Can you work these out from the model? Positions are in its coordinate system, mm. Face numbers are marked on the shaded views. A direction names the side the tool comes from. Round coordinates to 2 decimals unless told otherwise and drop trailing zeros. Loops run counter-clockwise (first coordinate to the right, second up) from the corner with the lowest first, then second, coordinate; pieces in that order, holes last.
from build123d import *

# Parameters (mm, degrees)
BOSS_EXTRUDE1_DEPTH                 = 8
SKETCH1_3_R                         = 10.5
SKETCH1_3_R_2                       = 4.5
BOSS_EXTRUDE2_DEPTH                 = 4
BOSS_EXTRUDE3_DEPTH                 = 8
CUT_EXTRUDE1_DEPTH                  = 4
DRAFT1_ANGLE                        = 1
DRAFT2_ANGLE                        = 30
CUT_EXTRUDE2_REACH                  = 100.996
CUT_EXTRUDE2_END_RADIUS             = 7.571153535
CUT_EXTRUDE2_START                  = -30
CUT_EXTRUDE2_DIRECTION_2_REACH      = 100.996
CUT_EXTRUDE2_DIRECTION_2_END_RADIUS = 7.571153535


with BuildPart() as part:
    # Sketch1 → Boss-Extrude1 (new body)
    with BuildSketch(Plane.XY):
        with BuildLine():
            Line((-2.665163662, 3.723158213), (-6.165163662, 3.723158213))
            Line((-6.165163662, 3.723158213), (-6.165163662, 3.223158213))
            Line((-6.165163662, 3.223158213), (-6.020826094, 2.973158213))
            Line((-6.020826094, 2.973158213), (-6.165163662, 2.723158213))
            Line((-6.165163662, 2.723158213), (-6.020826094, 2.473158213))
            Line((-6.020826094, 2.473158213), (-6.165163662, 2.223158213))
            Line((-6.165163662, 2.223158213), (-6.020826094, 1.973158213))
            Line((-6.020826094, 1.973158213), (-6.165163662, 1.723158213))
            Line((-6.165163662, 1.723158213), (-6.020826094, 1.473158213))
            Line((-6.020826094, 1.473158213), (-6.165163662, 1.223158213))
            Line((-6.165163662, 1.223158213), (-6.020826094, 0.973158213))
            Line((-6.020826094, 0.973158213), (-6.165163662, 0.723158213))
            Line((-6.165163662, 0.723158213), (-6.020826094, 0.473158213))
            Line((-6.020826094, 0.473158213), (-6.165163662, 0.223158213))
            Line((-6.165163662, 0.223158213), (-6.020826094, -0.026841787))
            Line((-6.020826094, -0.026841787), (-6.165163662, -0.276841787))
            Line((-6.165163662, -0.276841787), (-6.020826094, -0.526841787))
            Line((-6.020826094, -0.526841787), (-6.165163662, -0.776841787))
            Line((-6.165163662, -0.776841787), (-6.020826094, -1.026841787))
            Line((-6.020826094, -1.026841787), (-6.165163662, -1.276841787))
            Line((-6.165163662, -1.276841787), (-6.020826094, -1.526841787))
            Line((-6.020826094, -1.526841787), (-6.165163662, -1.776841787))
            Line((-6.165163662, -1.776841787), (-6.020826094, -2.026841787))
            Line((-6.020826094, -2.026841787), (-6.165163662, -2.276841787))
            Line((-6.165163662, -2.276841787), (-6.020826094, -2.526841787))
            Line((-6.020826094, -2.526841787), (-6.165163662, -2.776841787))
            Line((-6.165163662, -2.776841787), (-6.020826094, -3.026841787))
            Line((-6.020826094, -3.026841787), (-6.165163662, -3.276841787))
            Line((-6.165163662, -3.276841787), (-6.020826094, -3.526841787))
            Line((-6.020826094, -3.526841787), (-6.165163662, -3.776841787))
            Line((-6.165163662, -3.776841787), (-6.020826094, -4.026841787))
            Line((-6.020826094, -4.026841787), (-6.165163662, -4.276841787))
            Line((-6.165163662, -4.276841787), (-6.020826094, -4.526841787))
            Line((-6.020826094, -4.526841787), (-6.165163662, -4.776841787))
            Line((-6.165163662, -4.776841787), (-6.020826094, -5.026841787))
            Line((-6.020826094, -5.026841787), (-6.165163662, -5.276841787))
            Line((-6.165163662, -5.276841787), (-6.020826094, -5.526841787))
            Line((-6.020826094, -5.526841787), (-6.165163662, -5.776841787))
            Line((-6.165163662, -5.776841787), (-6.020826094, -6.026841787))
            Line((-6.020826094, -6.026841787), (-6.165163662, -6.276841787))
            Line((-6.165163662, -6.276841787), (-6.020826094, -6.526841787))
            Line((-6.020826094, -6.526841787), (-6.165163662, -6.776841787))
            Line((-6.165163662, -6.776841787), (-6.020826094, -7.026841787))
            Line((-6.020826094, -7.026841787), (-6.165163662, -7.276841787))
            Line((-6.165163662, -7.276841787), (-6.020826094, -7.526841787))
            Line((-6.020826094, -7.526841787), (-6.165163662, -7.776841787))
            Line((-6.165163662, -7.776841787), (-6.020826094, -8.026841787))
            Line((-6.020826094, -8.026841787), (-6.165163662, -8.276841787))
            Line((-6.165163662, -8.276841787), (-6.020826094, -8.526841787))
            Line((-6.020826094, -8.526841787), (-6.165163662, -8.776841787))
            Line((-6.165163662, -8.776841787), (-6.020826094, -9.026841787))
            Line((-6.020826094, -9.026841787), (-6.165163662, -9.276841787))
            Line((-6.165163662, -9.276841787), (-5.819249533, -10.684037163))
            Line((-5.819249533, -10.684037163), (-4.683707653, -11.584259383))
            Line((-4.683707653, -11.584259383), (-4.88515369, -13.019276771))
            Line((-4.88515369, -13.019276771), (-4.165163662, -14.276841787))
            Line((-4.165163662, -14.276841787), (-4.88515369, -15.534406803))
            Line((-4.88515369, -15.534406803), (-4.683707653, -16.969424191))
            Line((-4.683707653, -16.969424191), (-5.819249533, -17.869646411))
            Line((-5.819249533, -17.869646411), (-6.165163662, -19.276841787))
            Line((-6.165163662, -19.276841787), (-6.165163662, -32.776841787))
            ThreePointArc((-6.165163662, -32.776841787), (0.226831343, -34.946631714), (3.977057514, -40.559241813))
            Line((3.977057514, -40.559241813), (5.908909167, -40.041603723))
            Line((5.908909167, -40.041603723), (5.908909167, -25.025498714))
            Line((5.908909167, -25.025498714), (-2.665163662, 3.723158213))
        make_face()
    extrude(amount=-BOSS_EXTRUDE1_DEPTH)

    # Sketch1_3 → Boss-Extrude2 (add)
    with BuildSketch(Plane.XY):
        with Locations((-6.165163662, -43.276841787)):
            Circle(SKETCH1_3_R)
        with Locations((-6.165163662, -43.276841787)):
            Circle(SKETCH1_3_R_2, mode=Mode.SUBTRACT)
    extrude(amount=-BOSS_EXTRUDE2_DEPTH)

    # Sketch1_4 → Boss-Extrude3 (add)
    with BuildSketch(Plane.XY):
        with BuildLine():
            Line((5.908909167, -46.512079851), (3.977057514, -45.994441761))
            ThreePointArc((3.977057514, -45.994441761), (0.520445963, -51.373299281), (-5.415163662, -53.75002182))
            Line((-5.415163662, -53.75002182), (-5.415163662, -62.75002182))
            Line((-5.415163662, -62.75002182), (5.908909167, -57.512079851))
            Line((5.908909167, -57.512079851), (5.908909167, -46.512079851))
        make_face()
    extrude(amount=-BOSS_EXTRUDE3_DEPTH)

    # Sketch2 → Cut-Extrude1 (cut)
    with BuildSketch(Plane.XY):
        with BuildLine():
            Line((-6.165163662, -19.276841787), (-6.165163662, -32.776841787))
            ThreePointArc((-6.165163662, -32.776841787), (-2.023276207, -26.026841787), (-6.165163662, -19.276841787))
        make_face()
    extrude(amount=-CUT_EXTRUDE1_DEPTH, mode=Mode.SUBTRACT)

    # Draft1
    draft1_faces = [part.faces().sort_by_distance(p)[0] for p in [
        (-4.462150227, -26.026841787, -4),
    ]]
    draft(draft1_faces, Plane(origin=(-6.165163662, 0, -8), x_dir=(0, -1, 0), z_dir=(-1, 0, 0)), DRAFT1_ANGLE)

    # Draft2
    draft2_faces = [part.faces().sort_by_distance(p)[0] for p in [
        (-4.462150227, -26.026841787, -3.97027379),
    ]]
    draft(draft2_faces, Plane(origin=(-6.165163662, 0, -8), x_dir=(0, -1, 0), z_dir=(-1, 0, 0)), DRAFT2_ANGLE)

    # Cut-Extrude2: up to this cylinder (the profile starts inside it)
    cut_extrude2_end = Plane(origin=(-9.594429741, -26.026841787, -6.821489), z_dir=(0, 0, 1)) * Cylinder(CUT_EXTRUDE2_END_RADIUS, 218.134307069, mode=Mode.PRIVATE)
    # Sketch3 → Cut-Extrude2 (cut, up to the surface)
    with BuildSketch(Plane(origin=(0, 3.723158213, 0), x_dir=(1, 0, 0), z_dir=(0, 1, 0)).offset(CUT_EXTRUDE2_START), mode=Mode.PRIVATE) as cut_extrude2_sk1:
        Polygon((-6.165163662, 4.464466094), (-2.629629756, 8), (-6.165163662, 8), align=None)
    cut_extrude2_tool1 = extrude(cut_extrude2_sk1.sketch, amount=CUT_EXTRUDE2_REACH, mode=Mode.PRIVATE) & cut_extrude2_end
    add(cut_extrude2_tool1.solids().sort_by_distance((-4.986652, -26.276842, -6.821489))[0], mode=Mode.SUBTRACT)

    # Cut-Extrude2 direction 2: up to this cylinder (the profile starts inside it)
    cut_extrude2_direction_2_end = Plane(origin=(-9.594429741, -26.026841787, -6.821489), z_dir=(0, 0, 1)) * Cylinder(CUT_EXTRUDE2_DIRECTION_2_END_RADIUS, 218.134307069, mode=Mode.PRIVATE)
    # Sketch3 → Cut-Extrude2 direction 2 (cut, up to the surface)
    with BuildSketch(Plane(origin=(0, 3.723158213, 0), x_dir=(1, 0, 0), z_dir=(0, 1, 0)).offset(CUT_EXTRUDE2_START), mode=Mode.PRIVATE) as cut_extrude2_direction_2_sk1:
        Polygon((-6.165163662, 4.464466094), (-2.629629756, 8), (-6.165163662, 8), align=None)
    cut_extrude2_direction_2_tool1 = extrude(cut_extrude2_direction_2_sk1.sketch, amount=-CUT_EXTRUDE2_DIRECTION_2_REACH, mode=Mode.PRIVATE) & cut_extrude2_direction_2_end
    add(cut_extrude2_direction_2_tool1.solids().sort_by_distance((-4.986652, -26.276842, -6.821489))[0], mode=Mode.SUBTRACT)

    # Sweep1: sweep along a path in Sketch5
    with BuildLine() as sweep1_path:  # in the path sketch's own coordinates; laid on its plane below (add() does not lay a ready-made edge on the line's plane)
        add(Edge.make_bspline(
            [(0.223551669, -60.141837986), (21.749513364, -111.274227055), (24.236934906, -103.098193166), (21.841154622, -151.61274391)],
            knots=[0, 0, 0, 0, 1, 1, 1, 1], degree=3))
    # Sketch4 → Sweep1 (sweep)
    with BuildSketch(Plane(origin=(22.955106723, -49.62737309, 0), x_dir=(0.9076099917812164, 0.419814367094434, 0), z_dir=(0.41981436709443404, -0.9076099917812165, 0))):
        with BuildLine():
            Line((-27.545509922, -1), (-22.545509922, -1))
            ThreePointArc((-22.545509922, -1), (-19.545509922, -4), (-22.545509922, -7))
            Line((-22.545509922, -7), (-27.545509922, -7))
            ThreePointArc((-27.545509922, -7), (-30.545509922, -4), (-27.545509922, -1))
        make_face()
    sweep(path=Plane.XY.offset(-4) * sweep1_path.line)

    # Sweep3: sweep along a path in Sketch5_3
    with BuildLine() as sweep3_path:  # in the path sketch's own coordinates; laid on its plane below (add() does not lay a ready-made edge on the line's plane)
        add(Edge.make_bspline(
            [(0.223551669, -60.141837986), (21.749513364, -111.274227055), (24.236934906, -103.098193166), (21.841154622, -151.61274391)],
            knots=[0, 0, 0, 0, 1, 1, 1, 1], degree=3))
    # Sketch13 → Sweep3 (sweep)
    with BuildSketch(Plane(origin=(-2.2035554, -151.26246633, 0), x_dir=(0.9998939070612703, -0.014566215079688138, 0), z_dir=(-0.014566215079688138, -0.9998939070612703, 0))):
        with BuildLine():
            Line((21.547261266, -10), (26.547261266, -10))
            ThreePointArc((26.547261266, -10), (32.547261266, -4), (26.547261266, 2))
            Line((26.547261266, 2), (21.547261266, 2))
            ThreePointArc((21.547261266, 2), (15.547261266, -4), (21.547261266, -10))
        make_face()
    sweep(path=Plane.XY.offset(-4) * sweep3_path.line)


solid = part.part
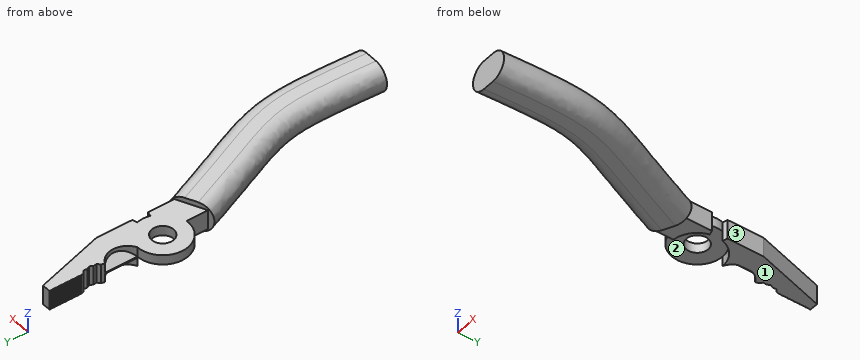
(1) For the marked faces 1, 2 and 3, which set-ups out of +Z, -Z, +X, -X, +Y, -Y let a thin tool reach every point of the face, with its end or its side?
Worked answers:
face 1: -Z, +X, -X, +Y
face 2: -Z, -X
face 3: +Z, -Z, +X, +Y
(2) Will these pins go through, and if not, where does the flat tip stop? P1, Ø9, axis at x = 2.5, y = -52, coming from the -Z side; P2, Ø6.5, axis at x = -2.5, y = -46, coming from the -Z side; P3, Ø1.5, axis at x = 13, y = -132.5, coming from the -Z side; P4, Ø4, axis at y = -54, z = -3, coming from the +X side.
Worked answers:
P1: stops at z = -8
P2: stops at z = -4
P3: passes through
P4: stops at x = 5.91
(3) If we section it at A-A, the plane y = -26.5: List the corners of the cut face in (x, z) for me, then the cut area to 3 significant figures.
Worked answers:
outline: (-6.17, -4.46) - (-2.63, -8) - (5.91, -8) - (5.91, 0) - (-2.04, 0) - (-2.04, -1.62) - (-6.17, -4) - close
area: 78.8 mm2
(4) If I drill on line 1 (X direction, y = -26, z = -3.5); line 2 (Z direction, x = -15, y = -48.5); line 3 (X direction, y = -128.5, z = -0.25), over which ranges is the centre line in solid material (lowest first)?
Worked answers:
line 1: x = -5.3 to 5.91
line 2: z = -4 to 0
line 3: x = 15.4 to 29.76
